CAD build for the part. Positions are in the model's coordinates, mm. A direction names the side the tool comes from. Round coordinates to 2 decimals unless told otherwise and drop trailing zeros. Order: outer loops, then holes, each group sorted by start corner. A loop starts at its lowest first (then second) coordinate and runs counter-clockwise, first axis right, second up. Notation, with made-up numbers: (20, 26.25) - (78, 26.25) arc R21 ccw to (78, 32.25) - close; hole circle Ø4 at (-37.75, -14.5). An arc over 180 degrees is marked (long way). Use one line per item in the form item = value. Start each with the question number.
Autodesk Inventor part; units mm, degrees
ref_plane "YZ Plane" through (0, 0, 0) normal (1, 0, 0) x (0, 1, 0)
ref_plane "XZ Plane" through (0, 0, 0) normal (0, 1, 0) x (-1, 0, 0)
ref_plane "XY Plane" through (0, 0, 0) normal (0, 0, 1) x (1, 0, 0)
sketch "スケッチ1" plane through (0, 0, 0) normal (0, 0, 1) x (1, 0, 0)
  line L0 (-17, -16) -> (17, -16) construction
  line L1 (17, -16) -> (17, 16) construction
  line L2 (17, 16) -> (-17, 16) construction
  line L3 (-17, 16) -> (-17, -16) construction
  line L4 (-17, -16) -> (17, 16) construction
  line L5 (17, -16) -> (-17, 16) construction
  line L6 (-17, 7.1) -> (-17, 16)
  line L7 (-17, 16) -> (17, 16)
  line L8 (17, 16) -> (17, 7.1)
  line L9 (-17, 5) -> (-22, 5)
  line L10 (-22, 5) -> (-22, -5)
  line L11 (-22, -5) -> (-17, -5)
  line L12 (17, 5) -> (22, 5)
  line L13 (22, 5) -> (22, -5)
  line L14 (22, -5) -> (17, -5)
  line L15 (-17, -7.1) -> (-17, -16)
  line L16 (-17, -16) -> (17, -16)
  line L17 (17, -16) -> (17, -7.1)
  arc A0 (-17, 5) -> (-17, 7.1) centre (-17, 6.05) ccw
  arc A1 (-17, -7.1) -> (-17, -5) centre (-17, -6.05) ccw
  arc A2 (17, 7.1) -> (17, 5) centre (17, 6.05) ccw
  arc A3 (17, -5) -> (17, -7.1) centre (17, -6.05) ccw
  line L18 (0, 0) -> (-17, 0) construction
  line L19 (0, 0) -> (0, 16) construction
  dimension "d87" = 32
  dimension "d88" = 1.05
  dimension "d89" = 5
  dimension "d90" = 11
  dimension "d91" = 34
extrude "押し出し1" add sketch "スケッチ1" along normal blind 5
sketch "スケッチ2" plane through (0, 0, 5) normal (0, 0, 1) x (1, 0, 0)
  line L0 (-17, 16) -> (-17, 7.1)
  line L1 (17, 7.1) -> (17, 16)
  line L2 (-28.2886, 18.8938) -> (-17, 18.8938)
  line L3 (-17, 18.8938) -> (-17, -23.6662)
  line L4 (-17, -23.6662) -> (-28.2886, -23.6662)
  line L5 (-28.2886, -23.6662) -> (-28.2886, 18.8938)
  line L6 (17, 13.565) -> (34.37, 13.565)
  line L7 (34.37, 13.565) -> (34.37, -20.2305)
  line L8 (34.37, -20.2305) -> (17, -20.2305)
  line L9 (17, -20.2305) -> (17, 13.565)
  point P0 (0, 0)
extrude "押し出し2" cut sketch "スケッチ2" against normal blind 2.5
sketch "スケッチ3" plane through (17, -16, 0) normal (1, 0, 0) x (0, 0, -1)
  line L0 (0, 0) -> (-5, 0)
  line L1 (-5, 11) -> (-5, 21) construction
  line L2 (-5, 16) -> (0, 16) construction
  point P0 (-2.5, 4)
  point P1 (-2.5, 28)
  point P2 (-2.5, 0)
  dimension "d96" = 4
hole "穴1" at (17, -12, 2.5) at (17, 12, 2.5) direction (-1, 0, 0) diameter 2.459 depth 2.5
mirror "ミラー1" about plane through (0, 0, 0) normal (1, 0, 0) of "穴1"
sketch "スケッチ4" plane through (0, 0, 5) normal (0, 0, 1) x (1, 0, 0)
  line L0 (-17, -16) -> (17, -16)
  line L1 (17, -16) -> (17, -7.1)
  line L2 (10, 12) -> (-10, 12) construction
  line L3 (-10, 12) -> (-10, -12) construction
  line L4 (-10, -12) -> (10, -12) construction
  line L5 (10, -12) -> (10, 12) construction
  line L6 (10, 12) -> (-10, -12) construction
  line L7 (-10, 12) -> (10, -12) construction
  circle A0 centre (0, 0) radius 12
  dimension "d104" = 4
  dimension "d105" = 7
extrude "押し出し3" cut sketch "スケッチ4" against normal blind 10
equation "\"d87\" = d3"
equation "\"d90\" = d77 + d82"
properties part number "コックピット_2_サブフレーム_6" material "アセタール樹脂、黒"
(1) Wall check: line 1 (Y direction, x = 15, z = 2.5); line 2 (Z direction, x = 16.25, y = 12); line 3 (Y direction, x = -16.2, z = 2.5). Give the ranges that are in metal, low to high. Write a range as [from, to].
(2) Flat gauge pins, fed straight in: P1, Ø3, axis at x = -19, z = 0.5, coming from the -Y side; P2, Ø0.7, axis at y = 12, z = 2, coming from the +X side; P3, Ø2, axis at y = -11.5, z = 3, coming from the -X side; P4, Ø2, axis at x = 5, y = 8, coming from the +Z side (3 decimals). Where does each tip first touch, or does it go through?
(3) Slice it at D-D (x = -5.5). Give the cut face in (y, z).
(4) Slice it at A-A (y = 0). Give the cut face in (x, z).
(5) Slice it at B-B (z = 4.4). Give the cut face in (x, y), and give its area (3 significant figures).
(6) Mould opens along Z. For faces 1 (the flat face through (17, -10.6, 2.5)), 2 (the flat face through (14.5, -12, 3)), 3 (the flat face through (-12, -3, 5)) say: pulls with the +Z half, pulls with the -Z half, needs draft (parallel to the pull), parting line crosses it, or undercut.
(7) Slice it at C-C (x = 10). Give the cut face in (y, z), and give its area (3 significant figures).
(8) Which spindle directions (+Z, -Z, +X, -X, +Y, -Y) get a long thin tool onto all of the face, cutting with end or side? Do faces 4 (the flat face through (20, -5, 1)), 5 (the flat face through (-17, 10, 2)), 6 (the flat face through (-20, 0, 2.5)), 7 (the flat face through (17, 0, 4)). Say none if no direction does.
Results list:
q1.line_1 = [-16, -13.23], [-10.77, 10.77], [13.23, 16]
q1.line_2 = [0, 1.27], [3.73, 5]
q1.line_3 = [-16, -13.23], [-10.77, -6.73], [-5.37, 5.37], [6.73, 10.77], [13.23, 16]
q2.P1 = -5
q2.P2 = 14.5
q2.P3 = -17
q2.P4 = through
q3.outline = (-16, 0) - (-10.67, 0) - (-10.67, 5) - (-16, 5) - close; (10.67, 0) - (16, 0) - (16, 5) - (10.67, 5) - close
q4.outline = (-22, 0) - (-12, 0) - (-12, 5) - (-17, 5) - (-17, 2.5) - (-22, 2.5) - close; (12, 0) - (22, 0) - (22, 2.5) - (17, 2.5) - (17, 5) - (12, 5) - close
q5.outline = (-17, -16) - (17, -16) - (17, -7.1) arc R1.05 cw to (17, -5) - (17, 5) arc R1.05 cw to (17, 7.1) - (17, 16) - (-17, 16) - (-17, 7.1) arc R1.05 cw to (-17, 5) - (-17, -5) arc R1.05 cw to (-17, -7.1) - close; hole circle Ø24 at (0, 0)
q5.area = 629 mm²
q6.face_1 = needs draft
q6.face_2 = undercut
q6.face_3 = pulls with the +Z half
q7.outline = (-16, 0) - (-6.63, 0) - (-6.63, 5) - (-16, 5) - close; (6.63, 0) - (16, 0) - (16, 5) - (6.63, 5) - close
q7.area = 93.7 mm²
q8.face_4 = +Z, -Z, +X, -Y
q8.face_5 = +Z, -Z, -X, +Y
q8.face_6 = +Z, -X, +Y, -Y
q8.face_7 = +Z, +X, +Y, -Y
